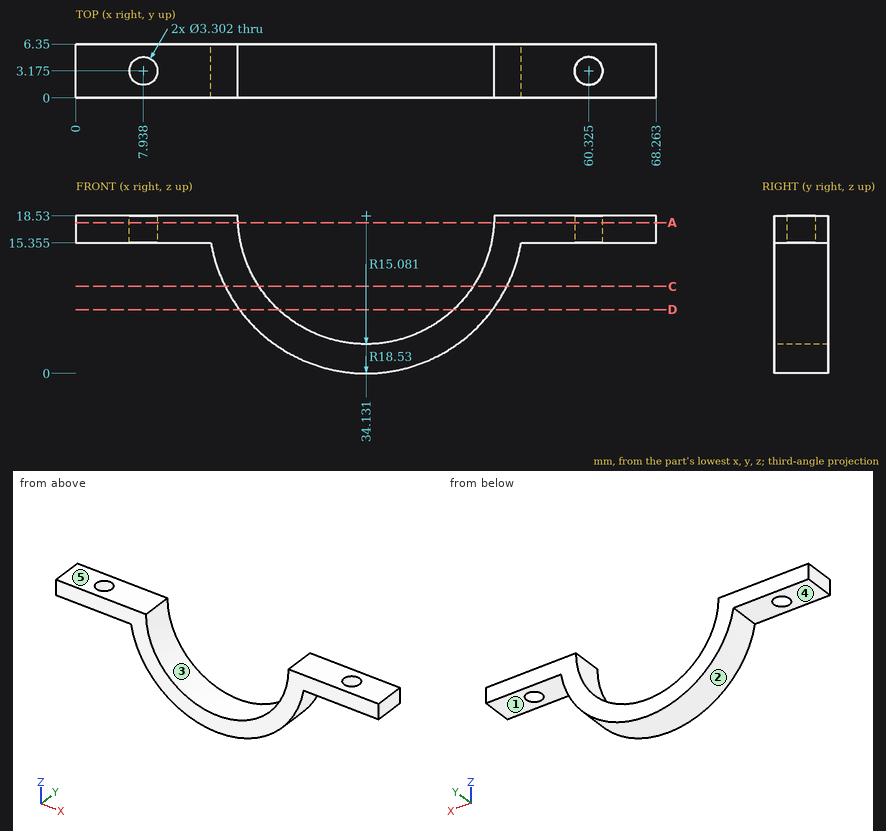
Study the drawing (mm; zero at the part's minimum x, y, z) and answer. A direction names the side the tool comes from. Give positions to 0.01 mm unless a question says otherwise; leave off trailing zeros. Write each loop counter-clockwise with the first axis right and the second up, starting at its lowest first coordinate (ties: lowest second). Pieces come first, ordered by that corner, then holes. Notation, with made-up numbers: (-38.75, 41.5) - (4.25, 41.5) arc R12 cw to (4.25, 60.5) - close; hole circle Ø11 at (-10.75, 43.5). An arc over 180 degrees is marked (long way). Use CSV: the item, a comma, the result in double quotes. Start each with the question number.
(1) Find section A-A (z = 17.75). Count the separate pieces of the cut face and the enclosed holes in it, plus the area to 3 significant figures.
(2) Find section C-C (z = 10.25). Give the vertices of the cut face in (x, y).
(3) For the marked faces 4 and 5, determine the directions among +Z, -Z, +X, -X, +Y, -Y from which every point of the face is accessible in a straight line to the end or side of a thin tool.
(4) Find section D-D (z = 7.5). Give the vertices of the cut face in (x, y).
(5) Given P1, Ø3, axis at x = 61, y = 2.5, coming from the -Z side (1 decimal); P2, Ø2, axis at x = 27.5, y = 2, coming from the -Z side, each flat-ended and moving along its own axis, determine where each tip first touches the part or whether it passes through.
(6) Determine the mould class of the marked faces 1, 2 and 3 for opening direction X: +X half, -X half, draft (parallel to the pull), parting line (faces both ways), or undercut.
(7) Consider line 1 along Z through (x, y) = (13.5, 5) (1 decimal); line 2 along Z through (x, y) = (34, 0.5); line 3 along X through (y, z) = (2.5, 12) (1 decimal). Determine where each line is inside the solid, lowest interval first.
Findings below:
1,separate pieces,"2"
1,enclosed holes,"2"
1,area,"225 mm2"
2,outline,"(17.55, 0) - (21.53, 0) - (21.53, 6.35) - (17.55, 6.35) - close; (46.74, 0) - (50.71, 0) - (50.71, 6.35) - (46.74, 6.35) - close"
3,face 4,"-Z, -X, +Y, -Y"
3,face 5,"+Z, +X, -X, +Y, -Y"
4,outline,"(19.24, 0) - (23.85, 0) - (23.85, 6.35) - (19.24, 6.35) - close; (44.42, 0) - (49.02, 0) - (49.02, 6.35) - (44.42, 6.35) - close"
5,P1,"z = 15.4"
5,P2,"z = 0.88"
6,face 1,"draft"
6,face 2,"parting line"
6,face 3,"undercut"
7,line 1,"15.4 to 18.5"
7,line 2,"0 to 3.45"
7,line 3,"16.8 to 20.5, 47.7 to 51.5"
